Autodesk Fusion 360 part; units mm, degrees
sketch "Esquisse1" plane through (0, 0, 0) normal (0, 0, 1) x (1, 0, 0)
  line L0 (75, -125) -> (-75, -125) construction
  line L1 (-75, -125) -> (-75, 125) construction
  line L2 (-75, 125) -> (75, 125) construction
  line L3 (75, 125) -> (75, -125) construction
  line L4 (75, -125) -> (-75, 125) construction
  line L5 (-75, -125) -> (75, 125) construction
  line L6 (-75, 125) -> (75, 125) construction
  line L7 (75, 125) -> (75, 136) construction
  line L8 (75, 136) -> (-75, 136) construction
  line L9 (-75, 136) -> (-75, 125) construction
  line L10 (-75, 136) -> (-75, 126)
  line L11 (-75, 126) -> (-65, 126)
  line L12 (-65, 126) -> (-65, -101)
  line L13 (-65, -101) -> (-75, -101)
  line L14 (-75, -101) -> (-75, -125)
  line L15 (-75, -125) -> (0, -125)
  line L16 (0, -125) -> (0, -120)
  line L17 (0, -120) -> (0, 136)
  line L18 (-75, 136) -> (0, 136)
  line L19 (75, 136) -> (0, 136)
  line L20 (75, 136) -> (75, 125) construction
  line L21 (0, -120) -> (0, 136)
  line L22 (0, -125) -> (0, -120)
  line L23 (75, -101) -> (75, -125)
  line L24 (75, -125) -> (0, -125)
  line L25 (65, -101) -> (75, -101)
  line L26 (75, -125) -> (75, 125) construction
  line L27 (75, 126) -> (65, 126)
  line L28 (75, 136) -> (75, 126)
  line L29 (65, 126) -> (65, -101)
  dimension "d1" = 150
  dimension "d2" = 250
  dimension "d3" = 11
  dimension "d4" = 10
  dimension "d5" = 10
  dimension "d6" = 24
extrude "Extrusion1" add sketch "Esquisse1" along normal blind 10
Can you work these out from the model? Positions are in its coordinate system, mm. A direction names the side the tool comes from. Coordinates: 2 decimals unless noted, no trailing zeros. Loops run counter-clockwise (first coordinate to the right, second up) from the corner with the lowest first, then second, coordinate; pieces in that order, holes last. Notation, with made-up numbers: (74, 53.5) -> (101, 53.5) arc R15 cw to (101, 78.5) -> close; hole circle Ø7 at (36.25, 75). An arc over 180 degrees is marked (long way). Put each result on its own line as item: value. Start each with the question number.
Q1. If I drill on line 1 (X direction, y = 44, z = 5.5), over which ranges is the centre line in solid material (lowest first)? Write a range as [from, to].
Q2. Thinking about a two-plate mould opening in Y: for faces 1 (the face through (-1, 7, 10)), 2 (the face through (-1, -125, 5)), 3 (the face through (70, 126, 5)), which applies, pulls with the +Y half, pulls with the -Y half, needs draft (parallel to the pull), parting line crosses it, or undercut?
Q3. For faces 4 (the face through (-70, 126, 5)), 5 (the face through (65, 14, 5)), 6 (the face through (75, -113, 5)), which set-ups out of +Z, -Z, +X, -X, +Y, -Y let a thin tool reach every point of the face, with its end or its side?
Q4. I want a section at A-A (z = 5). Write out the boundary of the cut face in (x, y), plus the area to 3 significant figures.
Q5. I want a section at B-B (y = 106). Write out the boundary of the cut face in (x, z).
Q6. I'm going to push a flat-ended pin straight in: P1, Ø3, axis at x = 26, y = -32, coming from the -Z side. Where does the tip first touch, or does it pass through?
Taken from the geometry:
1. line 1: x = [-65, 65]
2. face 1: needs draft
2. face 2: pulls with the -Y half
2. face 3: undercut
3. face 4: +Z, -Z, -X
3. face 5: +Z, -Z, +X
3. face 6: +Z, -Z, +X, +Y, -Y
4. outline: (-75, -125) -> (75, -125) -> (75, -101) -> (65, -101) -> (65, 126) -> (75, 126) -> (75, 136) -> (-75, 136) -> (-75, 126) -> (-65, 126) -> (-65, -101) -> (-75, -101) -> close
4. area: 34,600 mm2
5. outline: (-65, 0) -> (65, 0) -> (65, 10) -> (-65, 10) -> close
6. P1: stops at z = 0
